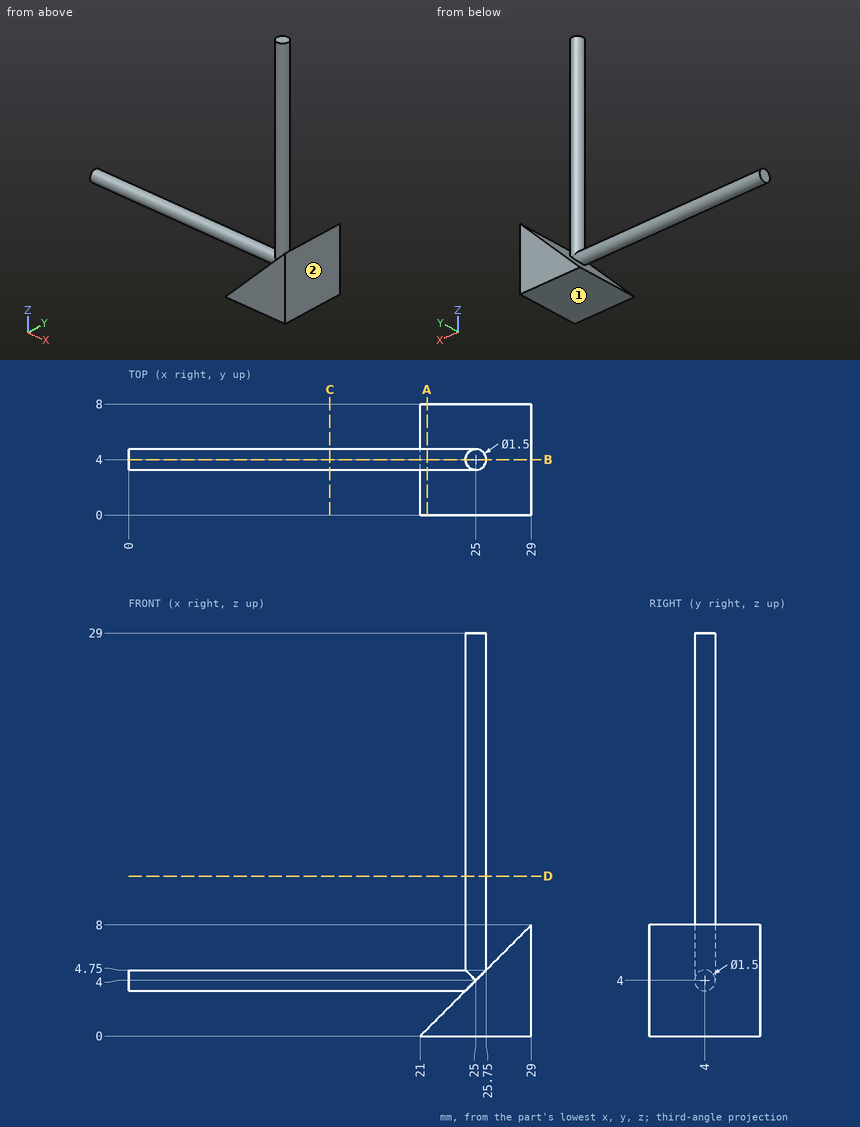
Drawing for the job (mm, zero at the part's lowest x, y, z). Give positions to 0.01 mm unless a question says otherwise; leave off trailing zeros. Write each loop counter-clockwise with the first axis right and the second up, starting at its lowest first coordinate (ties: lowest second). Pieces come first, ordered by that corner, then holes. Notation, with made-up numbers: (7.25, -14) - (36.25, -14) arc R23 ccw to (36.25, 12) - close; hole circle Ø6 at (22.5, 65.25). An arc over 180 degrees is marked (long way). Answer as CSV lines item,"result".
Q1. Band-saw the part on A-A (x = 21.5). Give the cut face in (y, z), and give its area (3 significant figures).
Result set:
outline,"(0, 0) - (8, 0) - (8, 0.5) - (0, 0.5) - close; circle Ø1.5 at (4, 4)"
area,"5.77 mm²"
Q2. Pull direction X, two halves, no side cores. Call the marked faces 1 and 2: released by +X, released by -X, zero draft, split by the parting line, or undercut.
Result set:
face 1,"zero draft"
face 2,"released by +X"
Q3. Band-saw the part on C-C (x = 14.5). Give the cut face in (y, z), and give its area (3 significant figures).
Result set:
outline,"circle Ø1.5 at (4, 4)"
area,"1.77 mm²"
Q4. Flat gauge pins, fed straight in: pin 1 Ø4 at (y, z) = (6.5, 21.5) entering from +X; pin 2 Ø2 at (x, y) = (7.5, 1) entering from +Z; pin 3 Ø8 at (x, z) = (25, 16.5) entering from +Y; pin 4 Ø3 at (y, z) = (5.5, 14) entering from +X. Where does each tip first touch, or does it go through?
Result set:
pin 1,"x = 25.56"
pin 2,"through"
pin 3,"y = 4.75"
pin 4,"x = 25.75"
Q5. Drill centre lines: line 1 (Y direction, x = 25, z = 26.5); line 2 (X direction, y = 4.25, z = 7.5); line 3 (Z direction, x = 22.75, y = 1.5). Where is each one in solid material? Low to high. Write a range as from..to.
Result set:
line 1,"3.25..4.75"
line 2,"24.29..25.71, 28.5..29"
line 3,"0..1.75"
Q6. Band-saw the part on B-B (y = 4). Give the cut face in (x, z).
Result set:
outline,"(0, 3.25) - (24.25, 3.25) - (21, 0) - (29, 0) - (29, 8) - (25.75, 4.75) - (25.75, 29) - (24.25, 29) - (24.25, 4.75) - (0, 4.75) - close"
Q7. Band-saw the part on D-D (z = 11.5). Give the cut face in (x, y), and give its area (3 significant figures).
Result set:
outline,"circle Ø1.5 at (25, 4)"
area,"1.77 mm²"
